Can you work these out from the model? Positions are in its coordinate system, mm. Face numbers are marked on the shaded views. Coordinates: 2 decimals unless noted, no trailing zeros. Write each loop counter-clockwise with the first axis right and the second up, starting at its lowest first coordinate (ties: lowest second). Pieces come first, ordered by that corner, then holes.
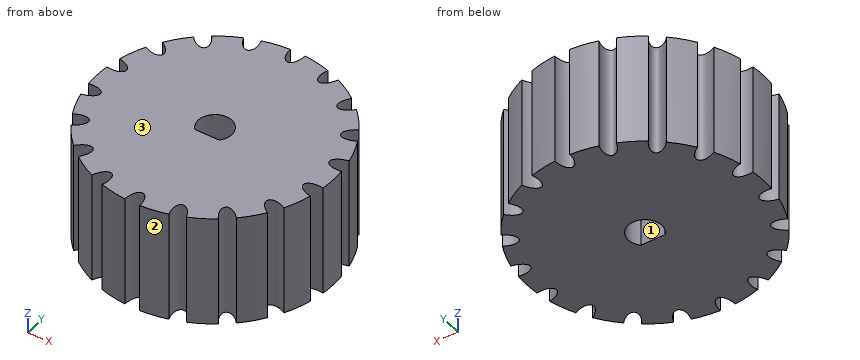
```python
from build123d import *

# Parameters (mm, degrees)
SKETCH_1_R               = 15.91549431
EXTRUDE_1_DEPTH          = 15
CUT_EXTRUDE_1_DEPTH      = 15
SKETCH_3_RX              = 2
SKETCH_3_RY              = 1
CUT_EXTRUDE_2_DEPTH      = 15
PATTERN_CIRCULAR_1_COUNT = 18


with BuildPart() as part:
    # Эскиз1 → Бобышка-Вытянуть1 (new body)
    with BuildSketch(Plane.XY):
        Circle(SKETCH_1_R)
    extrude(amount=EXTRUDE_1_DEPTH)

    # Эскиз2 → Вырез-Вытянуть1 (cut)
    with BuildSketch(Plane.XY.offset(15)):
        with BuildLine():
            Line((1.630950643, -1.55), (-1.630950643, -1.55))
            ThreePointArc((-1.630950643, -1.55), (0, 2.25), (1.630950643, -1.55))
        make_face()
    extrude(amount=-CUT_EXTRUDE_1_DEPTH, mode=Mode.SUBTRACT)

    # Эскиз3 → Вырез-Вытянуть2 (cut)
    with BuildSketch(Plane.XY.offset(15)):
        with Locations(Location((0.125778317, 15.914997296), (0, 0, 90))):
            Ellipse(SKETCH_3_RX, SKETCH_3_RY)
    cut_extrude_2 = extrude(amount=-CUT_EXTRUDE_2_DEPTH, mode=Mode.SUBTRACT)

    # Круговой массив1: Вырез-Вытянуть2 ×18 about axis
    pattern_circular_1_axis = Axis((0, 0, 15), (0, 0, 1))
    for i in range(1, PATTERN_CIRCULAR_1_COUNT):
        add(cut_extrude_2.rotate(pattern_circular_1_axis, i * 360 / PATTERN_CIRCULAR_1_COUNT), mode=Mode.SUBTRACT)


solid = part.part
```
1. If we section it at B-B, the plane x = -8: List the corners of the cut face in (y, z) for me, plus the area to 3 significant figures.
2. I'm going to push flat-ended pins straight in: P1, Ø5, axis at y = -5.5, z = 5, coming from the +X side; P2, Ø3, axis at y = 6, z = 10, coming from the -X side; P3, Ø5, axis at x = -3.5, z = 8, coming from the +Y side. Where does each tip first touch, or does it pass through?
3. If I drill on L1, parallel to X at y = 0, z = 3.5; L2, parallel to Y at x = 14.5, z = 2.75; L3, parallel to Y at x = 13, z = 7, over which ranges is the centre line in solid material (lowest first)?
4. If we section it at C-C, the plane x = -3: List the corners of the cut face in (y, z) for me, plus the area to 3 significant figures.
5. If we section it at A-A, the plane y = 1: List the corners of the cut face in (x, z) for me.
6. We'd pull the mould along X, two halves only. Please class the marked faces 1, 2 and 3: released by +X, released by -X, zero draft, split by the parting line, or undercut.
Answers:
1. outline: (-13.76, 0) - (13.76, 0) - (13.76, 15) - (-13.76, 15) - close
1. area: 413 mm2
2. P1: stops at x = 15.44
2. P2: stops at x = -15.27
2. P3: stops at y = 15.88
3. L1: x = -15.92 to -2.25, 2.25 to 15.92
3. L2: y = -6.56 to -3.56, -1.91 to 1.68, 3.29 to 6.56
3. L3: y = -9.18 to -8.8, -6.76 to 6.53, 8.49 to 9.18
4. outline: (-15.63, 0) - (15.63, 0) - (15.63, 15) - (-15.63, 15) - close
4. area: 469 mm2
5. outline: (-15.88, 0) - (-2.02, 0) - (-2.02, 15) - (-15.88, 15) - close; (2.02, 0) - (15.88, 0) - (15.88, 15) - (2.02, 15) - close
6. face 1: undercut
6. face 2: released by +X
6. face 3: zero draft
